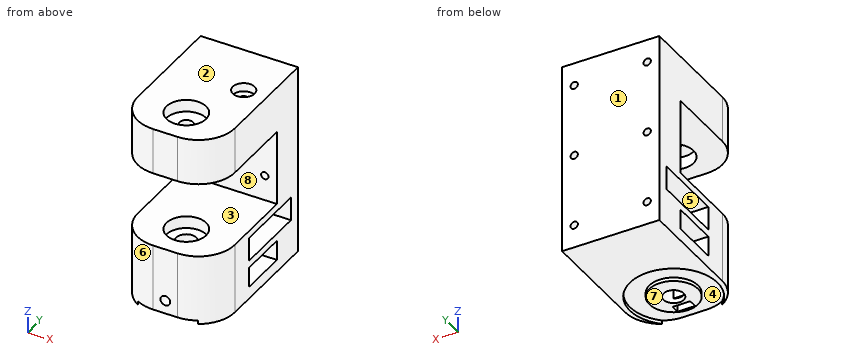
Autodesk Inventor part; units mm, degrees
ref_plane "YZ Plane" through (0, 0, 0) normal (1, 0, 0) x (0, 1, 0)
ref_plane "XZ Plane" through (0, 0, 0) normal (0, 1, 0) x (-1, 0, 0)
ref_plane "XY Plane" through (0, 0, 0) normal (0, 0, 1) x (1, 0, 0)
sketch "Sketch1" plane through (0, 0, 0) normal (0, 1, 0) x (-1, 0, 0)
  line L0 (20, 34.5) -> (-20, 34.5)
  line L1 (-20, 34.5) -> (-20, 15.5)
  line L2 (-20, 15.5) -> (20, 15.5)
  line L3 (20, 15.5) -> (20, 34.5)
  line L4 (20, -15.5) -> (-20, -15.5)
  line L5 (-20, -15.5) -> (-20, -44.5)
  line L6 (-20, -44.5) -> (20, -44.5)
  line L7 (20, -44.5) -> (20, -15.5)
  point P0 (0, 0)
  dimension "d0" = 31
  dimension "d1" = 19
  dimension "d2" = 40
  dimension "d3" = 20
  dimension "d4" = 29
  dimension "d50" = 15.5
sketch "Sketch1 outline for Extrusion1" plane through (0, 0, 0) normal (0, 1, 0) x (-1, 0, 0)
  line L0 (20, -15.5) -> (-20, -15.5)
  line L1 (20, -44.5) -> (20, -15.5)
  line L2 (-20, -44.5) -> (20, -44.5)
  line L3 (-20, -15.5) -> (-20, -44.5)
  line L4 (20, 34.5) -> (-20, 34.5)
  line L5 (20, 15.5) -> (20, 34.5)
  line L6 (-20, 15.5) -> (20, 15.5)
  line L7 (-20, 34.5) -> (-20, 15.5)
extrude "Extrusion1" add sketch "Sketch1 outline for Extrusion1" along normal blind 45
sketch "Sketch2" plane through (20, 0, -44.5) normal (0, 0, -1) x (-1, 0, 0)
  circle A0 centre (20, 15) radius 8.125
  line L0 (0, 0) -> (40, 0)
  circle A1 centre (20, 15) radius 2.75
  point P0 (20, 0)
  point P1 (20, 0)
  dimension "d7" = 16.25
  dimension "d8" = 15
  dimension "d9" = 5.5
sketch "Sketch2 outline for Extrusion2" plane through (20, 0, -44.5) normal (0, 0, -1) x (-1, 0, 0)
  circle A0 centre (20, 15) radius 2.75
extrude "Extrusion2" cut sketch "Sketch2 outline for Extrusion2" against normal blind 274.75
sketch "Sketch3" plane through (0, 45, 0) normal (0, 1, 0) x (1, 0, 0)
  line L0 (20, -34.5) -> (20, -15.5)
  line L1 (-20, 44.5) -> (-20, 15.5)
  line L2 (20, -34.5) -> (-20, -34.5)
  line L3 (-20, -34.5) -> (-20, 44.5)
  line L4 (-20, 44.5) -> (20, 44.5)
  line L5 (20, 44.5) -> (20, -34.5)
  point P0 (0, 0)
sketch "Sketch3 outline for Extrusion3" plane through (0, 45, 0) normal (0, 1, 0) x (1, 0, 0)
  line L0 (-20, -34.5) -> (20, -34.5)
  line L1 (-20, 15.5) -> (-20, -34.5)
  line L2 (-20, 44.5) -> (-20, 15.5)
  line L3 (20, 44.5) -> (-20, 44.5)
  line L4 (20, -15.5) -> (20, 44.5)
  line L5 (20, -34.5) -> (20, -15.5)
extrude "Extrusion3" add sketch "Sketch3 outline for Extrusion3" along normal blind 15
sketch "Sketch4" plane through (-20, 0, -44.5) normal (-1, 0, 0) x (0, 0, 1)
  line L0 (5, 55) -> (26, 55)
  line L1 (26, 55) -> (26, 25)
  line L2 (26, 25) -> (5, 25)
  line L3 (5, 25) -> (5, 55)
  line L4 (0, 0) -> (0, 60)
  line L5 (29, 0) -> (29, 45)
  line L6 (0, 60) -> (79, 60)
  line L7 (0, 0) -> (29, 0)
  line L8 (13.25, 55) -> (16.25, 55)
  line L9 (16.25, 55) -> (16.25, 25)
  line L10 (16.25, 25) -> (13.25, 25)
  line L11 (13.25, 25) -> (13.25, 55)
  line L12 (5, 55) -> (13.25, 55)
  line L13 (13.25, 45) -> (5, 45)
  point P0 (44.5, 0)
  dimension "d14" = 5
  dimension "d15" = 3
  dimension "d16" = 5
  dimension "d18" = 3
  dimension "d19" = 9.75
  dimension "d45" = 25
sketch "Sketch4 outline for Extrusion4" plane through (-20, 0, -44.5) normal (-1, 0, 0) x (0, 0, 1)
  line L0 (26, 25) -> (26, 55)
  line L1 (16.25, 25) -> (26, 25)
  line L2 (16.25, 55) -> (16.25, 25)
  line L3 (26, 55) -> (16.25, 55)
  line L4 (13.25, 45) -> (5, 45)
  line L5 (13.25, 25) -> (13.25, 45)
  line L6 (5, 25) -> (13.25, 25)
  line L7 (5, 45) -> (5, 25)
extrude "Extrusion4" cut sketch "Sketch4 outline for Extrusion4" against normal blind 100
sketch "Sketch5" plane through (20, 0, -44.5) normal (0, 0, -1) x (-1, 0, 0)
  circle A0 centre (20, 15) radius 2.75
  circle A1 centre (20, 15) radius 4.15
  line L0 (17.935418, 11.4) -> (22.064582, 11.4)
  point P0 (20, 0)
  dimension "d22" = 8.3
  dimension "d24" = 3.6
sketch "Sketch5 outline for Extrusion5" plane through (20, 0, -44.5) normal (0, 0, -1) x (-1, 0, 0)
  line L0 (17.935418, 11.4) -> (22.064582, 11.4)
  arc A0 (22.064582, 11.4) -> (17.935418, 11.4) centre (20, 15) ccw
  circle A1 centre (20, 15) radius 2.75
extrude "Extrusion5" cut sketch "Sketch5 outline for Extrusion5" against normal blind 25
sketch "Sketch6" plane through (20, 0, -44.5) normal (0, 0, -1) x (-1, 0, 0)
  line L0 (16.375, 9.5) -> (23.625, 9.5)
  line L1 (23.625, 9.5) -> (23.625, 6)
  line L2 (23.625, 6) -> (16.375, 6)
  line L3 (16.375, 6) -> (16.375, 9.5)
  line L4 (0, 0) -> (40, 0)
  circle A0 centre (20, 15) radius 2.75
  point P0 (20, 0)
  point P1 (20, 0)
  dimension "d27" = 3.5
  dimension "d28" = 7.25
  dimension "d29" = 3.625
  dimension "d30" = 5.5
sketch "Sketch6 outline for Extrusion6" plane through (20, 0, -44.5) normal (0, 0, -1) x (-1, 0, 0)
  line L0 (16.375, 9.5) -> (16.375, 6)
  line L1 (23.625, 9.5) -> (16.375, 9.5)
  line L2 (23.625, 6) -> (23.625, 9.5)
  line L3 (16.375, 6) -> (23.625, 6)
extrude "Extrusion6" cut sketch "Sketch6 outline for Extrusion6" against normal blind 23
sketch "Sketch7" plane through (0, 0, 0) normal (0, -1, 0) x (1, 0, 0)
  circle A0 centre (0, -37.5) radius 2
  point P0 (0, 0)
  dimension "d33" = 4
  dimension "d34" = 37.5
sketch "Sketch7 outline for Extrusion7" plane through (0, 0, 0) normal (0, -1, 0) x (1, 0, 0)
  circle A0 centre (0, -37.5) radius 2
extrude "Extrusion7" cut sketch "Sketch7 outline for Extrusion7" against normal blind 15.5
sketch "Sketch8" plane through (-20, 0, -15.5) normal (0, 0, 1) x (1, 0, 0)
  circle A0 centre (20, 15) radius 2.75
  circle A1 centre (20, 15) radius 8.15
  point P0 (20, 0)
  dimension "d37" = 16.3
sketch "Sketch8 outline for Extrusion8" plane through (-20, 0, -15.5) normal (0, 0, 1) x (1, 0, 0)
  circle A0 centre (20, 15) radius 8.15
  circle A1 centre (20, 15) radius 2.75
extrude "Extrusion8" cut sketch "Sketch8 outline for Extrusion8" against normal blind 5
sketch "Sketch9" plane through (-20, 0, 34.5) normal (0, 0, 1) x (1, 0, 0)
  circle A0 centre (20, 15) radius 2.75
  circle A1 centre (20, 15) radius 8.15
  point P0 (20, 0)
sketch "Sketch9 outline for Extrusion9" plane through (-20, 0, 34.5) normal (0, 0, 1) x (1, 0, 0)
  circle A0 centre (20, 15) radius 8.15
  circle A1 centre (20, 15) radius 2.75
extrude "Extrusion9" cut sketch "Sketch9 outline for Extrusion9" against normal blind 5
sketch "Sketch10" plane through (20, 0, 15.5) normal (0, 0, -1) x (-1, 0, 0)
  circle A0 centre (20, 15) radius 2.75
  circle A1 centre (20, 15) radius 8.15
  point P0 (20, 0)
sketch "Sketch10 outline for Extrusion10" plane through (20, 0, 15.5) normal (0, 0, -1) x (-1, 0, 0)
  circle A0 centre (20, 15) radius 8.15
  circle A1 centre (20, 15) radius 2.75
extrude "Extrusion10" cut sketch "Sketch10 outline for Extrusion10" against normal blind 5
fillet "Fillet1" radius 15 4 edges at (-20, 0, -30) (-20, 0, 25) (20, 0, 25) (20, 0, -30)
sketch "Sketch11" plane through (0, 60, 0) normal (0, 1, 0) x (1, 0, 0)
  line L0 (-15, -25) -> (15, -25)
  line L1 (15, -25) -> (15, 35)
  line L2 (15, 35) -> (-15, 35)
  line L3 (-15, 35) -> (-15, -25)
  circle A0 centre (-15, -25) radius 1.5
  circle A1 centre (-15, 35) radius 1.5
  circle A2 centre (15, 35) radius 1.5
  circle A3 centre (15, -25) radius 1.5
  circle A4 centre (-15, 5) radius 1.5
  circle A5 centre (15, 5) radius 1.5
  point P0 (0, 0)
  dimension "d46" = 60
  dimension "d47" = 30
  dimension "d48" = 15
  dimension "d49" = 25
  dimension "d51" = 3
  dimension "d52" = 3
  dimension "d53" = 3
  dimension "d54" = 3
  dimension "d55" = 3
  dimension "d56" = 3
sketch "Sketch11 outline for Extrusion11" plane through (0, 60, 0) normal (0, 1, 0) x (1, 0, 0)
  circle A0 centre (-15, 35) radius 1.5
  circle A1 centre (15, -25) radius 1.5
  circle A2 centre (15, 5) radius 1.5
  circle A3 centre (-15, -25) radius 1.5
  circle A4 centre (15, 35) radius 1.5
  circle A5 centre (-15, 5) radius 1.5
extrude "Extrusion11" cut sketch "Sketch11 outline for Extrusion11" against normal blind 15
sketch "Sketch12" plane through (20, 60, -44.5) normal (0, 0, -1) x (-1, 0, 0)
  arc A0 (22.064582, -48.6) -> (17.935418, -48.6) centre (20, -45) ccw
  circle A1 centre (20, -45) radius 4.15
  point P0 (20, -60)
  point P1 (17.935418, -48.6)
sketch "Sketch12 outline for Extrusion12" plane through (20, 60, -44.5) normal (0, 0, -1) x (-1, 0, 0)
  arc A0 (17.935418, -48.6) -> (22.064582, -48.6) centre (20, -45) ccw
  arc A1 (22.064582, -48.6) -> (17.935418, -48.6) centre (20, -45) ccw
extrude "Extrusion12" cut sketch "Sketch12 outline for Extrusion12" against normal blind 2
sketch "Sketch13" plane through (20, 60, -44.5) normal (0, 0, -1) x (-1, 0, 0)
  arc A0 (22.064582, -48.6) -> (17.935418, -48.6) centre (20, -45) ccw
  circle A1 centre (20, -45) radius 10
  line L0 (20, -35) -> (40, -35)
  line L1 (40, -35) -> (0, -35)
  line L2 (0, -45) -> (0, 0)
  circle A2 centre (20, -45) radius 4.15
  arc A3 (0, -45) -> (15, -60) centre (15, -45) ccw
  line L3 (15, -60) -> (25, -60)
  arc A4 (25, -60) -> (40, -45) centre (25, -45) ccw
  line L4 (40, -45) -> (40, 0)
  line L5 (0, 0) -> (40, 0)
  line L6 (0, -45) -> (0, 0)
  line L7 (23.625, -50.5) -> (23.625, -54)
  line L8 (23.625, -54) -> (16.375, -54)
  line L9 (16.375, -54) -> (16.375, -50.5)
  line L10 (16.375, -50.5) -> (23.625, -50.5)
  circle A5 centre (20, -45) radius 18
  point P0 (20, -60)
  point P1 (40, -35)
  point P2 (17.935418, -48.6)
  point P3 (7.6, -58.047605)
  point P4 (34.96663, -35)
  point P5 (32.4, -58.047605)
  dimension "d61" = 20
  dimension "d64" = 36
sketch "Sketch13 outline for Extrusion13" plane through (20, 60, -44.5) normal (0, 0, -1) x (-1, 0, 0)
  circle A0 centre (20, -45) radius 4.15
  line L0 (23.625, -50.5) -> (16.375, -50.5)
  line L1 (23.625, -54) -> (23.625, -50.5)
  line L2 (16.375, -54) -> (23.625, -54)
  line L3 (16.375, -50.5) -> (16.375, -54)
  arc A1 (32.4, -58.047605) -> (7.6, -58.047605) centre (20, -45) ccw
  arc A2 (25, -60) -> (32.4, -58.047605) centre (25, -45) ccw
  arc A3 (7.6, -58.047605) -> (15, -60) centre (15, -45) ccw
  line L4 (15, -60) -> (25, -60)
  circle A4 centre (20, -45) radius 10
extrude "Extrusion13" cut sketch "Sketch13 outline for Extrusion13" against normal blind 1.5
sketch "Sketch14" plane through (-20, 60, 34.5) normal (0, 0, 1) x (1, 0, 0)
  circle A0 centre (30.565457, -22.342305) radius 4.5
  circle A1 centre (20, -45) radius 2.75
  circle A2 centre (30.565457, -22.342305) radius 1.5
  line L0 (20, -45) -> (20, 2.624244)
  line L1 (20, 2.624244) -> (20, -45)
  line L2 (30.565457, -22.342305) -> (20, -45)
  point P0 (20, -60)
  dimension "d65" = 25
  dimension "d66" = 9
  dimension "d67" = 3
  dimension "d72" = 25
sketch "Sketch14 outline for Extrusion14" plane through (-20, 60, 34.5) normal (0, 0, 1) x (1, 0, 0)
  circle A0 centre (30.565457, -22.342305) radius 1.5
extrude "Extrusion14" cut sketch "Sketch14 outline for Extrusion14" against normal blind 10
sketch "Sketch14 outline for Extrusion15" plane through (-20, 60, 34.5) normal (0, 0, 1) x (1, 0, 0)
  circle A0 centre (30.565457, -22.342305) radius 4.5
  circle A1 centre (30.565457, -22.342305) radius 1.5
extrude "Extrusion15" cut sketch "Sketch14 outline for Extrusion15" against normal blind 3.5
properties part number "Gimbal_1"
Check sheet for the modelled part. Datum: model origin and axes. Units: mm. Face numbers are marked on the shaded views. A direction names the side the tool comes from. Round coordinates to 2 decimals unless told otherwise and drop trailing zeros. Order: outer loops, then holes, each group sorted by start corner. A loop starts at its lowest first (then second) coordinate and runs counter-clockwise, first axis right, second up.
(1) Cross-section at C-C, the plane z = -5. Enter the section's corners in (x, y), and give its area (3 significant figures).
(2) Go/stop test with flat-tipped pins: P1, Ø4.5, axis at x = 0, y = 15, coming from the +Z side; P2, Ø5, axis at x = 15, z = -35, coming from the +Y side; P3, Ø5, axis at x = -8.5, z = -22, coming from the -Y side; P4, Ø10, axis at x = 0, y = 15, coming from the +Z side. Record where each tip stops, or that it passes through.
(3) Cross-section at B-B, the plane x = -15. State how many separate pieces and enclosed holes the cut face has, and give its area (3 significant figures).
(4) Draft check along Z on the marked faces 1, 2 and 3. Enter one of: pulls with the +Z half, pulls with the -Z half, needs draft (parallel to the pull), parting line crosses it, or undercut.
(5) Cross-section at D-D, the plane z = -37.5. Enter the section's corners in (x, y) (3 decimals).
(6) Access from +Z, -Z, +X, -X, +Y, -Y to the whole of each face (thin tool, end or side, straight path). Record for the marked faces 4, 5, 6, 7 and 8.
(7) Cross-section at A-A, the plane z = -27. Enter the section's corners in (x, y) (3 decimals).
(8) Scan lines: probe 1 along Z at (x, y) = (0, 1.5); probe 2 along Z at (x, y) = (3.5, 31); probe 3 along Z at (x, y) = (-13, 41.5). Record each from-to range of solid material in increasing order.
Check sheet entries:
1. outline: (-20, 45) - (-16.5, 45) - (-16.5, 60) - (-20, 60) - close; (-13.5, 45) - (13.5, 45) - (13.5, 60) - (-13.5, 60) - close; (16.5, 45) - (20, 45) - (20, 60) - (16.5, 60) - close
1. area: 510 mm2
2. P1: passes through
2. P2: stops at y = 60
2. P3: stops at y = 0.03
2. P4: stops at z = 29.5
3. separate pieces: 2
3. enclosed holes: 1
3. area: 2,540 mm2
4. face 1: needs draft
4. face 2: pulls with the +Z half
4. face 3: undercut
5. outline: (-20, 15) arc R15 ccw to (-5, 0) - (-2, 0) - (-2, 6) - (-3.625, 6) - (-3.625, 9.5) - (-2, 9.5) - (-2, 11.4) - (-2.065, 11.4) arc R4.15 cw (long way) to (2.065, 11.4) - (2, 11.4) - (2, 9.5) - (3.625, 9.5) - (3.625, 6) - (2, 6) - (2, 0) - (5, 0) arc R15 ccw to (20, 15) - (20, 25) - (-20, 25) - close; (-20, 45) - (20, 45) - (20, 60) - (-20, 60) - close
6. face 4: -Z
6. face 5: +X, -X
6. face 6: +Z, -Z, -X, -Y
6. face 7: -Z, +X, -X, +Y, -Y
6. face 8: +X, -X, -Y
7. outline: (-20, 15) arc R15 ccw to (-5, 0) - (5, 0) arc R15 ccw to (20, 15) - (20, 25) - (-20, 25) - close; (-20, 55) - (20, 55) - (20, 60) - (-20, 60) - close; hole (-3.625, 6) - (3.625, 6) - (3.625, 9.5) - (-3.625, 9.5) - close; hole (-2.065, 11.4) - (2.065, 11.4) arc R4.15 ccw (long way) to start
8. probe 1: z = -43 to -39.5, -35.5 to -15.5, 15.5 to 34.5
8. probe 2: z = -43 to -39.5, -31.25 to -28.25, -18.5 to -15.5, 15.5 to 34.5
8. probe 3: z = -44.5 to -39.5, -31.25 to -28.25, -18.5 to -15.5, 15.5 to 34.5
